```python
from build123d import *

# Parameters (mm, degrees)
SALIENTE_EXTRUIR1_DEPTH = 1
REDONDEO1_R             = 0.05
CORTAR_EXTRUIR1_DEPTH   = 1
REDONDEO2_R             = 0.05
CROQUIS3_R              = 0.05
CORTAR_EXTRUIR2_DEPTH   = 9.502352647
CORTAR_EXTRUIR3_DEPTH   = 0.2


with BuildPart() as part:
    # Croquis1 → Saliente-Extruir1 (new body)
    with BuildSketch(Plane(origin=(0, 0, 0), x_dir=(1, 0, 0), z_dir=(0, 1, 0))):
        with BuildLine():
            Line((0, 0), (0, 1.328125))
            Line((0, 1.328125), (6, 1.328125))
            ThreePointArc((6, 1.328125), (6.283772234, 1.476808298), (6.6, 1.528125))
            Line((6.6, 1.528125), (7.8, 1.528125))
            Line((7.8, 1.528125), (7.8, 1.328125))
            Line((7.8, 1.328125), (8, 1.328125))
            Line((8, 1.328125), (8, -1.171875))
            Line((8, -1.171875), (7.8, -1.171875))
            Line((7.8, -1.171875), (7.8, -1.371875))
            Line((7.8, -1.371875), (6.6, -1.371875))
            ThreePointArc((6.6, -1.371875), (6.283772234, -1.320558298), (6, -1.171875))
            Line((6, -1.171875), (0, -1.171875))
            Line((0, -1.171875), (0, 0))
        make_face()
    extrude(amount=SALIENTE_EXTRUIR1_DEPTH)

    # Redondeo1
    redondeo1_edges = [part.edges().sort_by_distance(p)[0] for p in [
        (8, 0, -0.078125),
        (6.283772234, 0, -1.476808298),
        (3, 0, -1.328125),
        (0, 0, -0.078125),
        (6.283772234, 0, 1.320558298),
        (0, 0.5, 1.171875),
        (6, 0.5, 1.171875),
        (3, 0, 1.171875),
        (3, 1, -1.328125),
        (6.283772234, 1, -1.476808298),
        (8, 1, -0.078125),
        (6.283772234, 1, 1.320558298),
        (3, 1, 1.171875),
        (0, 1, -0.078125),
        (7.2, 0, 1.371875),
        (7.2, 0, -1.528125),
        (7.2, 1, -1.528125),
        (7.2, 1, 1.371875),
        (7.8, 0.5, 1.371875),
        (8, 0.5, 1.171875),
        (6, 0.5, -1.328125),
    ]]
    fillet(redondeo1_edges, radius=REDONDEO1_R)

    # Croquis2 → Cortar-Extruir1 (cut)
    with BuildSketch(Plane(origin=(0, 1, 0), x_dir=(1, 0, 0), z_dir=(0, 1, 0))):
        with BuildLine():
            Line((7.3, -0.771875), (7.3, 0.928125))
            ThreePointArc((7.3, 0.928125), (7, 1.228125), (6.7, 0.928125))
            Line((6.7, 0.928125), (6.7, -0.771875))
            ThreePointArc((6.7, -0.771875), (7, -1.071875), (7.3, -0.771875))
        make_face()
    extrude(amount=-CORTAR_EXTRUIR1_DEPTH, mode=Mode.SUBTRACT)

    # Redondeo2
    redondeo2_edges = [part.edges().sort_by_distance(p)[0] for p in [
        (7, 0, -1.228125),
        (7.3, 0, -0.078125),
        (7, 0, 1.071875),
        (6.7, 0, -0.078125),
        (7, 1, -1.228125),
        (6.7, 1, -0.078125),
        (7, 1, 1.071875),
        (7.3, 1, -0.078125),
    ]]
    fillet(redondeo2_edges, radius=REDONDEO2_R)

    # Croquis3 → Cortar-Extruir2 (cut, through all)
    with BuildSketch(Plane.XY.offset(1.171875)):
        with Locations((7.875, 0.500489471)):
            Circle(CROQUIS3_R)
        with Locations((0.15, 0.500489471)):
            Circle(CROQUIS3_R)
    extrude(amount=-CORTAR_EXTRUIR2_DEPTH, mode=Mode.SUBTRACT)

    # Croquis4 → Cortar-Extruir3 (cut)
    with BuildSketch(Plane(origin=(0, 1, 0), x_dir=(1, 0, 0), z_dir=(0, 1, 0))):
        Polygon((7.95, -0.071875), (7.75, -0.071875), (7.75, 0.078125), (7.95, 0.078125), (8.181877464, 0.078125), (8.181877464, -0.071875), align=None)
    extrude(amount=-CORTAR_EXTRUIR3_DEPTH, mode=Mode.SUBTRACT)


solid = part.part
```
Part model, mm, in its own coordinate system. A direction names the side the tool comes from. Round coordinates to 2 decimals unless told otherwise and drop trailing zeros. Order: outer loops, then holes, each group sorted by start corner. A loop starts at its lowest first (then second) coordinate and runs counter-clockwise, first axis right, second up. Notation, with made-up numbers: M 76.25,28 L 111.25,28 A28 ccw 111.25,67 Z; hole C 89,-11 d2. An arc over 180 degrees is marked long. Put each result on its own line as item: value. Start each with the question number.
1. Tool access for faces 4 (the face through (3.1, 0.5, 1.172)), 5 (the face through (6.7, 0.5, -0.1)), 6 (the face through (2.9, 0.5, -1.328)), 7 (the face through (4, 1, 0)), 8 (the face through (7.2, 0.5, 1.372)): list every direction of +Z, -Z, +X, -X, +Y, -Y with a clear straight run to the whole face (end or side of a thin tool).
2. Slice it at D-D on z = 1. State how many separate pieces and enclosed holes the cut face has, then the cut area to 3 significant figures.
3. Slice it at A-A on x = 7. List the corners of the cut face in (y, z), then the cut area to 3 significant figures.
4. Slice it at C-C on x = 4.75. List the corners of the cut face in (y, z), then the cut area to 3 significant figures.
5. Slice it at B-B on z = -0.5. List the corners of the cut face in (x, y) (3 decimals).
6. Drill centre lines: probe 1 along X at (y, z) = (0.65, -0.75); probe 2 along Z at (x, y) = (3, 0.5); probe 3 along Z at (x, y) = (6.5, 0.6). Where is each one in solid material? Low to high. Write a range as [from, to].
7. Two-plate mould, pull along X, no slides. Class faces 1 (the face through (7.2, 0.5, -1.528)), 2 (the face through (7.3, 0.5, -0.1)), 3 (the face through (0, 0.3, -0.1)): +X half, -X half, draft (parallel to the pull), parting line (faces both ways), or undercut.
Findings:
1. face 4: +Z, -X, +Y, -Y
1. face 5: +Y, -Y
1. face 6: -Z, -X, +Y, -Y
1. face 7: +Z, -Z, +X, -X, +Y
1. face 8: +Z, +X, -X, +Y, -Y
2. separate pieces: 2
2. enclosed holes: 2
2. area: 7.59 mm2
3. outline: M 0,-1.48 A0.05 ccw 0.05,-1.53 L 0.95,-1.53 A0.05 ccw 1,-1.48 L 1,-1.28 A0.05 ccw 0.95,-1.23 L 0.05,-1.23 A0.05 ccw 0,-1.28 Z; M 0,1.12 A0.05 ccw 0.05,1.07 L 0.95,1.07 A0.05 ccw 1,1.12 L 1,1.32 A0.05 ccw 0.95,1.37 L 0.05,1.37 A0.05 ccw 0,1.32 Z
3. area: 0.596 mm2
4. outline: M 0,-1.28 A0.05 ccw 0.05,-1.33 L 0.95,-1.33 A0.05 ccw 1,-1.28 L 1,1.12 A0.05 ccw 0.95,1.17 L 0.05,1.17 A0.05 ccw 0,1.12 Z
4. area: 2.50 mm2
5. outline: M 0,0.05 A0.05 ccw 0.05,0 L 6.65,0 A0.05 ccw 6.7,0.05 L 6.7,0.95 A0.05 ccw 6.65,1 L 0.05,1 A0.05 ccw 0,0.95 Z; M 7.3,0.05 A0.05 ccw 7.35,0 L 7.95,0 A0.05 ccw 8,0.05 L 8,0.95 A0.05 ccw 7.95,1 L 7.35,1 A0.05 ccw 7.3,0.95 Z; hole C 0.15,0.5 d0.1; hole C 7.875,0.5 d0.1
6. probe 1: [0, 6.7], [7.3, 8]
6. probe 2: [-1.33, 1.17]
6. probe 3: [-1.52, 1.37]
7. face 1: draft
7. face 2: undercut
7. face 3: -X half
